Model file for the job. Use its own axes, mm. Face numbers are marked on the shaded views. A direction names the side the tool comes from. Round coordinates to 2 decimals unless told otherwise and drop trailing zeros. Loops run counter-clockwise (first coordinate to the right, second up) from the corner with the lowest first, then second, coordinate; pieces in that order, holes last. Notation, with made-up numbers: (75.5, 57) - (102.5, 57) arc R26 ccw to (102.5, 82) - close; hole circle Ø10 at (61.5, -18). An arc over 180 degrees is marked (long way). Answer as a JSON object with one key per item and string values.
from build123d import *

# Parameters (mm, degrees)
SKETCH1_R            = 17
BOSS_EXTRUDE1_DEPTH  = 25
SKETCH1_3_R          = 19
BOSS_EXTRUDE2_DEPTH  = 8
BOSS_EXTRUDE3_DEPTH  = 15
SKETCH5_R            = 16
BOSS_EXTRUDE4_DEPTH  = 15
SKETCH6_R            = 17
BOSS_EXTRUDE5_DEPTH  = 5
BOSS_EXTRUDE6_DEPTH  = 15
SKETCH8_R            = 16
BOSS_EXTRUDE7_DEPTH  = 30
BOSS_EXTRUDE8_DEPTH  = 15
SKETCH10_R           = 17
BOSS_EXTRUDE9_DEPTH  = 2.5
BOSS_EXTRUDE10_DEPTH = 20
BOSS_EXTRUDE11_DEPTH = 20


with BuildPart() as part:
    # Sketch1 → Boss-Extrude1 (new body)
    with BuildSketch(Plane(origin=(0, 0, 0), x_dir=(0, 0, -1), z_dir=(1, 0, 0))):
        Circle(SKETCH1_R)
    extrude(amount=BOSS_EXTRUDE1_DEPTH)

    # Sketch1_3 → Boss-Extrude2 (add)
    with BuildSketch(Plane(origin=(0, 0, 0), x_dir=(0, 0, -1), z_dir=(1, 0, 0))):
        Circle(SKETCH1_3_R)
    extrude(amount=-BOSS_EXTRUDE2_DEPTH)

    # Sketch4 → Boss-Extrude3 (add)
    with BuildSketch(Plane.ZY.offset(8)):
        with BuildLine():
            ThreePointArc((-13.668094758, 40.943123461), (0, 46), (13.668094758, 40.943123461))
            ThreePointArc((13.668094758, 40.943123461), (33.683444249, 16.469257624), (44, -13.416407865))
            ThreePointArc((44, -13.416407865), (0, -46), (-44, -13.416407865))
            ThreePointArc((-44, -13.416407865), (-33.683444249, 16.469257624), (-13.668094758, 40.943123461))
        make_face()
    boss_extrude3 = extrude(amount=BOSS_EXTRUDE3_DEPTH)

    # Sketch5 → Boss-Extrude4 (add)
    with BuildSketch(Plane.ZY.offset(23)):
        with Locations((0, 25)):
            Circle(SKETCH5_R)
    boss_extrude4 = extrude(amount=BOSS_EXTRUDE4_DEPTH)

    # Mirror1: Boss-Extrude3, Boss-Extrude4 across plane
    add(boss_extrude3.mirror(Plane(origin=(-38, 25, 0), x_dir=(0, 0, 1), z_dir=(-1, 0, 0))))
    add(boss_extrude4.mirror(Plane(origin=(-38, 25, 0), x_dir=(0, 0, 1), z_dir=(-1, 0, 0))))

    # Sketch6 → Boss-Extrude5 (add)
    with BuildSketch(Plane.ZY.offset(68)):
        Circle(SKETCH6_R)
    extrude(amount=BOSS_EXTRUDE5_DEPTH)

    # Sketch7 → Boss-Extrude6 (add)
    with BuildSketch(Plane.ZY.offset(73)):
        with BuildLine():
            ThreePointArc((-13.668094758, -40.943123461), (0, -46), (13.668094758, -40.943123461))
            ThreePointArc((13.668094758, -40.943123461), (33.683444249, -16.469257624), (44, 13.416407865))
            ThreePointArc((44, 13.416407865), (0, 46), (-44, 13.416407865))
            ThreePointArc((-44, 13.416407865), (-33.683444249, -16.469257624), (-13.668094758, -40.943123461))
        make_face()
    extrude(amount=BOSS_EXTRUDE6_DEPTH)

    # Sketch8 → Boss-Extrude7 (add)
    with BuildSketch(Plane.ZY.offset(88)):
        with Locations((0, -25)):
            Circle(SKETCH8_R)
    extrude(amount=BOSS_EXTRUDE7_DEPTH)

    # Sketch9 → Boss-Extrude8 (add)
    with BuildSketch(Plane.ZY.offset(118)):
        with BuildLine():
            ThreePointArc((-13.668094758, -40.943123461), (0, -46), (13.668094758, -40.943123461))
            ThreePointArc((13.668094758, -40.943123461), (33.683444249, -16.469257624), (44, 13.416407865))
            ThreePointArc((44, 13.416407865), (0, 46), (-44, 13.416407865))
            ThreePointArc((-44, 13.416407865), (-33.683444249, -16.469257624), (-13.668094758, -40.943123461))
        make_face()
    extrude(amount=BOSS_EXTRUDE8_DEPTH)

    # Sketch10 → Boss-Extrude9 (add)
    with BuildSketch(Plane.ZY.offset(133)):
        Circle(SKETCH10_R)
    extrude(amount=BOSS_EXTRUDE9_DEPTH)

    # Mirror2: part across plane


with BuildPart() as part_1:
    add(part.part)
    add(part.part.mirror(Plane.ZY.offset(135.5)))

    # Sketch11 → Boss-Extrude10 (add)
    with BuildSketch(Plane(origin=(25, 0, 0), x_dir=(0, 0, -1), z_dir=(1, 0, 0))):
        Polygon((14.722431864, -8.5), (14.722431864, 8.5), (0, 17), (-14.722431864, 8.5), (-14.722431864, -8.5), (0, -17), align=None)
    extrude(amount=BOSS_EXTRUDE10_DEPTH)

    # Sketch12 → Boss-Extrude11 (add)
    with BuildSketch(Plane.ZY.offset(296)):
        Polygon((-14.722431864, -8.5), (0, -17), (14.722431864, -8.5), (14.722431864, 8.5), (0, 17), (-14.722431864, 8.5), align=None)
    extrude(amount=BOSS_EXTRUDE11_DEPTH)


solid = part_1.part
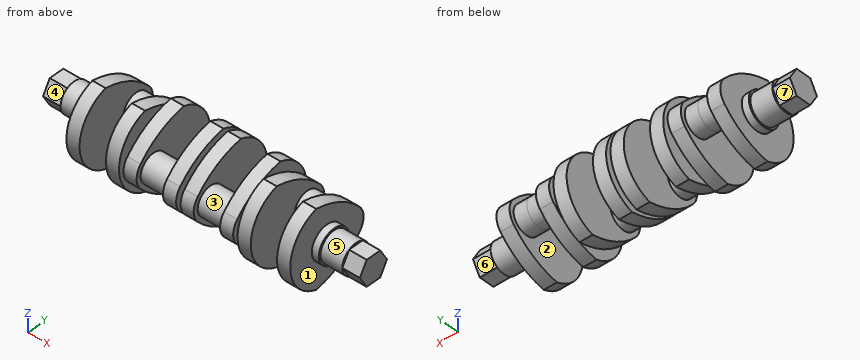
1) Slice it at A-A on z = -34.5. Count the separate pieces of the cut face and the enclosed holes in it, then the cut area to 3 significant figures.
Values follow:
{"separate pieces": "8", "enclosed holes": "0", "area": "5,450 mm²"}
2) Two-plate mould, pull along X, no slides. Class the marked faces 1, 2, 3 and 4: pulls with the +X half, pulls with the -X half, needs draft (parallel to the pull), parting line crosses it, or undercut.
Values follow:
{"face 1": "pulls with the +X half", "face 2": "undercut", "face 3": "undercut", "face 4": "needs draft"}
3) Probe probe 1 along X at (y, z) = (-15, 39); probe 2 along X at (y, z) = (28, 2.5); probe 3 along X at (y, z) = (10, -10). List the from-to ranges inside material, lowest first.
Values follow:
{"probe 1": "-263 to -248, -218 to -203, -68 to -53, -23 to -8", "probe 2": "-263 to -203, -198 to -183, -153 to -138, -133 to -118, -88 to -73, -68 to -8", "probe 3": "-316 to -248, -218 to -183, -153 to -118, -88 to -53, -23 to 45"}
4) Tool access for the marked faces 5, 6 and 7: list every direction of +Z, -Z, +X, -X, +Y, -Y with a clear straight run to the whole face (end or side of a thin tool).
Values follow:
{"face 5": "+X", "face 6": "-Z, +X, +Y", "face 7": "-Z, -X, +Y"}
5) Slice it at C-C on x = -291. List the corners of the cut face in (y, z), then the cut area to 3 significant figures.
Values follow:
{"outline": "circle Ø34 at (0, 0)", "area": "908 mm²"}
6) Drop flat-ended pins along their axis: P1, Ø0.7, axis at y = -0.5, z = 15.5, coming from the +X side; P2, Ø0.7, axis at y = -2.5, z = 16, coming from the -X side; P3, Ø12, axis at x = -5, y = -20, coming from the -Z side; P4, Ø5, axis at x = -26.5, z = -25.5, coming from the +Y side. Give the stop position or say it passes through.
Values follow:
{"P1": "x = 25", "P2": "x = -296", "P3": "z = -43.55", "P4": "through"}
